For this review, take the finished solid that the model builds, in its own axes (mm). A direction names the side the tool comes from. Coordinates: 2 decimals unless noted, no trailing zeros. Loops run counter-clockwise (first coordinate to the right, second up) from the corner with the lowest first, then second, coordinate; pieces in that order, holes last. Notation, with made-up numbers: M -19.5,-39 L 13.5,-39 A19 cw 13.5,-15 Z; hole C -23.5,-8 d2. An arc over 180 degrees is marked long. Put each result on its own line as item: value.
```python
from build123d import *

# Parameters (mm, degrees)
F0_W     = 50.8
F0_H     = 101.6
F0_W_2   = 44.45
F0_H_2   = 95.25
F1_DEPTH = 1524
F3_DEPTH = 173.228
F4_R     = 5.08


# Not quite as in the source:
# - a feature names something its author has since deleted; it is built from what else it names


with BuildPart() as f1:
    # F0 (on Front) → F1 (new body)
    with BuildSketch(Plane.XZ):
        with Locations((25.4, 50.8)):
            Rectangle(F0_W, F0_H)
        with Locations((25.4, 50.8)):
            Rectangle(F0_W_2, F0_H_2, mode=Mode.SUBTRACT)
    extrude(amount=F1_DEPTH)

    # F2 (on face) → F3 (cut)
    with BuildSketch(Plane.XY.offset(101.6)):
        Polygon((50.8, -1473.2), (0, -1524), (50.8, -1524), align=None)
    extrude(amount=-F3_DEPTH, mode=Mode.SUBTRACT)

    # F4
    f4_edges = [f1.edges().sort_by_distance(p)[0] for p in [
        (0, -762, 0),
        (50.8, -736.6, 0),
        (50.8, -736.6, 101.6),
        (0, -762, 101.6),
    ]]
    fillet(f4_edges, radius=F4_R)


solid = f1.part
```
(1) Add section B-B (z = 84). Write out the cut boundary in (x, y) (3 decimals), plus the area to 3 significant figures.
Determined:
outline: M 0,-1524 L 3.175,-1520.825 L 3.175,0 L 0,0 Z; M 47.625,-1476.375 L 50.8,-1473.2 L 50.8,0 L 47.625,0 Z
area: 9,520 mm^2
(2) Wall thickness on line 1 along Z through (x, y) = (39.5, -1448) (3 decimals); line 2 along X through (y, z) = (-586, 88) (3 decimals); line 3 along Z through (x, y) = (4, -749.5) (3 decimals): over which ranges is each line inside the solid? List them lowest first. Write a range as [from, to].
Determined:
line 1: z = [0, 3.175], [98.425, 101.6]
line 2: x = [0, 3.175], [47.625, 50.8]
line 3: z = [0.116, 3.175], [98.425, 101.484]
(3) Tool access review of faces 5 (the flat face through (50.8, -726, 50)), 6 (the flat face through (25, -750, 98.425)): name each direction out of +Z, -Z, +X, -X, +Y, -Y from which nothing blocks a thin tool from reaching the whole face with its end or side.
Determined:
face 5: +Z, -Z, +X, +Y, -Y
face 6: +Y, -Y
(4) Add section A-A (x = 25). Write out the cut boundary in (y, z) (3 decimals).
Determined:
outline: M -1499,0 L 0,0 L 0,3.175 L -1499,3.175 Z; M -1499,98.425 L 0,98.425 L 0,101.6 L -1499,101.6 Z
(5) Add section C-C (y = -110.5). Write out the cut boundary in (x, z) (3 decimals).
Determined:
outline: M 0,5.08 A5.08 ccw 5.08,0 L 45.72,0 A5.08 ccw 50.8,5.08 L 50.8,96.52 A5.08 ccw 45.72,101.6 L 5.08,101.6 A5.08 ccw 0,96.52 Z; hole M 3.175,3.175 L 47.625,3.175 L 47.625,98.425 L 3.175,98.425 Z
(6) Draft analysis for pull direction Z (two halves, no side actions). For faces 1 (the flat face through (0, -751, 50)), 2 (the flat face through (3.175, -750, 50)), 3 (the flat face through (47.625, -728, 50)), 4 (the flat face through (25, -749, 0)), state which applies: +Z half, -Z half, draft (parallel to the pull), parting line (faces both ways), or undercut.
Determined:
face 1: draft
face 2: undercut
face 3: undercut
face 4: -Z half
